Geometry check sheet. Reference: the model listing, model coordinates, mm. A direction names the side the tool comes from. Round coordinates to 2 decimals unless told otherwise and drop trailing zeros. Loops run counter-clockwise (first coordinate to the right, second up) from the corner with the lowest first, then second, coordinate; pieces in that order, holes last.
```python
from build123d import *

# Parameters (mm, degrees)
SKETCH_2_W      = 200
SKETCH_2_H      = 200
SKETCH_2_R      = 1.6
SKETCH_2_R_2    = 3
SKETCH_2_W_2    = 3
SKETCH_2_H_2    = 40
EXTRUDE_1_DEPTH = 3
FILLET_2_R      = 20


with BuildPart() as part:
    # 草图2 → 凸台-拉伸1 (new body)
    with BuildSketch(Plane(origin=(0, 0, 0), x_dir=(1, 0, 0), z_dir=(0, 1, 0))):
        Rectangle(SKETCH_2_W, SKETCH_2_H)
        with Locations(Location((-52.5, 52.5, 0), (0, 0, 270))):
            Circle(SKETCH_2_R, mode=Mode.SUBTRACT)
        with Locations(Location((-45.428932188, 45.428932188, 0), (0, 0, 270))):
            Circle(SKETCH_2_R, mode=Mode.SUBTRACT)
        with Locations(Location((-38.357864376, 38.357864376, 0), (0, 0, 270))):
            Circle(SKETCH_2_R, mode=Mode.SUBTRACT)
        with Locations(Location((52.5, 52.5, 0), (0, 0, 270))):
            Circle(SKETCH_2_R, mode=Mode.SUBTRACT)
        with Locations(Location((45.428932188, 45.428932188, 0), (0, 0, 270))):
            Circle(SKETCH_2_R, mode=Mode.SUBTRACT)
        with Locations(Location((38.357864376, 38.357864376, 0), (0, 0, 270))):
            Circle(SKETCH_2_R, mode=Mode.SUBTRACT)
        with Locations(Location((52.5, -52.5, 0), (0, 0, 270))):
            Circle(SKETCH_2_R, mode=Mode.SUBTRACT)
        with Locations(Location((45.428932188, -45.428932188, 0), (0, 0, 270))):
            Circle(SKETCH_2_R, mode=Mode.SUBTRACT)
        with Locations(Location((38.357864376, -38.357864376, 0), (0, 0, 270))):
            Circle(SKETCH_2_R, mode=Mode.SUBTRACT)
        with Locations(Location((-52.5, -52.5, 0), (0, 0, 270))):
            Circle(SKETCH_2_R, mode=Mode.SUBTRACT)
        with Locations(Location((-45.428932188, -45.428932188, 0), (0, 0, 270))):
            Circle(SKETCH_2_R, mode=Mode.SUBTRACT)
        with Locations(Location((-38.357864376, -38.357864376, 0), (0, 0, 270))):
            Circle(SKETCH_2_R, mode=Mode.SUBTRACT)
        with Locations(Location((0, 0, 0), (0, 0, 270))):
            Circle(SKETCH_2_R_2, mode=Mode.SUBTRACT)
        with BuildLine():
            Line((-60, 73.5), (60, 73.5))
            ThreePointArc((60, 73.5), (69, 82.5), (60, 91.5))
            Line((60, 91.5), (-60, 91.5))
            ThreePointArc((-60, 91.5), (-69, 82.5), (-60, 73.5))
        make_face(mode=Mode.SUBTRACT)
        with BuildLine():
            Line((-60, -73.5), (60, -73.5))
            ThreePointArc((60, -73.5), (69, -82.5), (60, -91.5))
            Line((60, -91.5), (-60, -91.5))
            ThreePointArc((-60, -91.5), (-69, -82.5), (-60, -73.5))
        make_face(mode=Mode.SUBTRACT)
        with Locations((74.942911166, 65)):
            Rectangle(SKETCH_2_W_2, SKETCH_2_H_2, mode=Mode.SUBTRACT)
        with Locations((87.942911166, 65)):
            Rectangle(SKETCH_2_W_2, SKETCH_2_H_2, mode=Mode.SUBTRACT)
        with Locations((74.942911166, -65)):
            Rectangle(SKETCH_2_W_2, SKETCH_2_H_2, mode=Mode.SUBTRACT)
        with Locations((87.942911166, -65)):
            Rectangle(SKETCH_2_W_2, SKETCH_2_H_2, mode=Mode.SUBTRACT)
        with Locations((-74.942911166, -65)):
            Rectangle(SKETCH_2_W_2, SKETCH_2_H_2, mode=Mode.SUBTRACT)
        with Locations((-87.942911166, -65)):
            Rectangle(SKETCH_2_W_2, SKETCH_2_H_2, mode=Mode.SUBTRACT)
        with Locations((-87.942911166, 65)):
            Rectangle(SKETCH_2_W_2, SKETCH_2_H_2, mode=Mode.SUBTRACT)
        with Locations((-74.942911166, 65)):
            Rectangle(SKETCH_2_W_2, SKETCH_2_H_2, mode=Mode.SUBTRACT)
        with BuildLine():
            Line((22.714466094, 23.428932188), (-22.714466094, 23.428932188))
            ThreePointArc((-22.714466094, 23.428932188), (-26.714466094, 27.428932188), (-22.714466094, 31.428932188))
            Line((-22.714466094, 31.428932188), (22.714466094, 31.428932188))
            ThreePointArc((22.714466094, 31.428932188), (26.714466094, 27.428932188), (22.714466094, 23.428932188))
        make_face(mode=Mode.SUBTRACT)
        with BuildLine():
            Line((22.714466094, 41.428932188), (-22.714466094, 41.428932188))
            ThreePointArc((-22.714466094, 41.428932188), (-26.714466094, 45.428932188), (-22.714466094, 49.428932188))
            Line((-22.714466094, 49.428932188), (22.714466094, 49.428932188))
            ThreePointArc((22.714466094, 49.428932188), (26.714466094, 45.428932188), (22.714466094, 41.428932188))
        make_face(mode=Mode.SUBTRACT)
        with BuildLine():
            Line((22.714466094, 59.428932188), (-22.714466094, 59.428932188))
            ThreePointArc((-22.714466094, 59.428932188), (-26.714466094, 63.428932188), (-22.714466094, 67.428932188))
            Line((-22.714466094, 67.428932188), (22.714466094, 67.428932188))
            ThreePointArc((22.714466094, 67.428932188), (26.714466094, 63.428932188), (22.714466094, 59.428932188))
        make_face(mode=Mode.SUBTRACT)
        with BuildLine():
            Line((22.714466094, -23.428932188), (-22.714466094, -23.428932188))
            ThreePointArc((-22.714466094, -23.428932188), (-26.714466094, -27.428932188), (-22.714466094, -31.428932188))
            Line((-22.714466094, -31.428932188), (22.714466094, -31.428932188))
            ThreePointArc((22.714466094, -31.428932188), (26.714466094, -27.428932188), (22.714466094, -23.428932188))
        make_face(mode=Mode.SUBTRACT)
        with BuildLine():
            Line((22.714466094, -41.428932188), (-22.714466094, -41.428932188))
            ThreePointArc((-22.714466094, -41.428932188), (-26.714466094, -45.428932188), (-22.714466094, -49.428932188))
            Line((-22.714466094, -49.428932188), (22.714466094, -49.428932188))
            ThreePointArc((22.714466094, -49.428932188), (26.714466094, -45.428932188), (22.714466094, -41.428932188))
        make_face(mode=Mode.SUBTRACT)
        with BuildLine():
            Line((22.714466094, -59.428932188), (-22.714466094, -59.428932188))
            ThreePointArc((-22.714466094, -59.428932188), (-26.714466094, -63.428932188), (-22.714466094, -67.428932188))
            Line((-22.714466094, -67.428932188), (22.714466094, -67.428932188))
            ThreePointArc((22.714466094, -67.428932188), (26.714466094, -63.428932188), (22.714466094, -59.428932188))
        make_face(mode=Mode.SUBTRACT)
        with BuildLine():
            Line((22.5, -12.5), (22.5, 12.5))
            ThreePointArc((22.5, 12.5), (25, 15), (27.5, 12.5))
            Line((27.5, 12.5), (27.5, -12.5))
            ThreePointArc((27.5, -12.5), (25, -15), (22.5, -12.5))
        make_face(mode=Mode.SUBTRACT)
        with BuildLine():
            Line((32.5, -17.5), (32.5, 17.5))
            ThreePointArc((32.5, 17.5), (35, 20), (37.5, 17.5))
            Line((37.5, 17.5), (37.5, -17.5))
            ThreePointArc((37.5, -17.5), (35, -20), (32.5, -17.5))
        make_face(mode=Mode.SUBTRACT)
        with BuildLine():
            Line((42.5, -22.5), (42.5, 22.5))
            ThreePointArc((42.5, 22.5), (45, 25), (47.5, 22.5))
            Line((47.5, 22.5), (47.5, -22.5))
            ThreePointArc((47.5, -22.5), (45, -25), (42.5, -22.5))
        make_face(mode=Mode.SUBTRACT)
        with BuildLine():
            Line((52.5, -27.5), (52.5, 27.5))
            ThreePointArc((52.5, 27.5), (55, 30), (57.5, 27.5))
            Line((57.5, 27.5), (57.5, -27.5))
            ThreePointArc((57.5, -27.5), (55, -30), (52.5, -27.5))
        make_face(mode=Mode.SUBTRACT)
        with BuildLine():
            Line((62.5, -32.5), (62.5, 32.5))
            ThreePointArc((62.5, 32.5), (65, 35), (67.5, 32.5))
            Line((67.5, 32.5), (67.5, -32.5))
            ThreePointArc((67.5, -32.5), (65, -35), (62.5, -32.5))
        make_face(mode=Mode.SUBTRACT)
        with BuildLine():
            Line((-22.5, -12.5), (-22.5, 12.5))
            ThreePointArc((-22.5, 12.5), (-25, 15), (-27.5, 12.5))
            Line((-27.5, 12.5), (-27.5, -12.5))
            ThreePointArc((-27.5, -12.5), (-25, -15), (-22.5, -12.5))
        make_face(mode=Mode.SUBTRACT)
        with BuildLine():
            Line((-32.5, -17.5), (-32.5, 17.5))
            ThreePointArc((-32.5, 17.5), (-35, 20), (-37.5, 17.5))
            Line((-37.5, 17.5), (-37.5, -17.5))
            ThreePointArc((-37.5, -17.5), (-35, -20), (-32.5, -17.5))
        make_face(mode=Mode.SUBTRACT)
        with BuildLine():
            Line((-42.5, -22.5), (-42.5, 22.5))
            ThreePointArc((-42.5, 22.5), (-45, 25), (-47.5, 22.5))
            Line((-47.5, 22.5), (-47.5, -22.5))
            ThreePointArc((-47.5, -22.5), (-45, -25), (-42.5, -22.5))
        make_face(mode=Mode.SUBTRACT)
        with BuildLine():
            Line((-52.5, -27.5), (-52.5, 27.5))
            ThreePointArc((-52.5, 27.5), (-55, 30), (-57.5, 27.5))
            Line((-57.5, 27.5), (-57.5, -27.5))
            ThreePointArc((-57.5, -27.5), (-55, -30), (-52.5, -27.5))
        make_face(mode=Mode.SUBTRACT)
        with BuildLine():
            Line((-62.5, -32.5), (-62.5, 32.5))
            ThreePointArc((-62.5, 32.5), (-65, 35), (-67.5, 32.5))
            Line((-67.5, 32.5), (-67.5, -32.5))
            ThreePointArc((-67.5, -32.5), (-65, -35), (-62.5, -32.5))
        make_face(mode=Mode.SUBTRACT)
        with BuildLine():
            Line((88.942911166, 30), (88.942911166, -30))
            ThreePointArc((88.942911166, -30), (81.442911166, -37.5), (73.942911166, -30))
            Line((73.942911166, -30), (73.942911166, 30))
            ThreePointArc((73.942911166, 30), (81.442911166, 37.5), (88.942911166, 30))
        make_face(mode=Mode.SUBTRACT)
        with BuildLine():
            Line((-88.942911166, 30), (-88.942911166, -30))
            ThreePointArc((-88.942911166, -30), (-81.442911166, -37.5), (-73.942911166, -30))
            Line((-73.942911166, -30), (-73.942911166, 30))
            ThreePointArc((-73.942911166, 30), (-81.442911166, 37.5), (-88.942911166, 30))
        make_face(mode=Mode.SUBTRACT)
    extrude(amount=EXTRUDE_1_DEPTH)

    # 圆角2
    fillet_2_edges = [part.edges().sort_by_distance(p)[0] for p in [
        (-100, 1.5, -100),
        (100, 1.5, -100),
        (100, 1.5, 100),
        (-100, 1.5, 100),
    ]]
    fillet(fillet_2_edges, radius=FILLET_2_R)


solid = part.part
```
1) Sectioned sample at B-B, the plane z = 0. State how many separate pieces and enclosed holes the cut face has, then the cut area to 3 significant figures.
Report:
separate pieces: 14
enclosed holes: 0
area: 342 mm2
2) Sectioned sample at A-A, the plane x = -65. Record the cut outline in (y, z).
Report:
outline: (0, -100) - (3, -100) - (3, -89.98) - (0, -89.98) - close; (0, -75.02) - (3, -75.02) - (3, -35) - (0, -35) - close; (0, 35) - (3, 35) - (3, 75.02) - (0, 75.02) - close; (0, 89.98) - (3, 89.98) - (3, 100) - (0, 100) - close
3) Access from +Z, -Z, +X, -X, +Y, -Y to the whole of each face (thin tool, end or side, straight path). Record for faces 1 (the face through (-94.297, 1.521, 93.986)), 2 (the face through (68.998, 1.479, 82.302)).
Report:
face 1: +Z, -X, +Y, -Y
face 2: +Y, -Y
4) Mould release check, pull along X, two halves, no side actions. Record for faces 3 (the face through (-24, 3, 21)), 4 (the face through (68.998, 1.479, -82.302)), 5 (the face through (93.986, 1.521, -94.297)): +X half, -X half, draft (parallel to the pull), parting line (faces both ways), or undercut.
Report:
face 3: draft
face 4: undercut
face 5: +X half
5) Gauge pin test, flat end, axial feed: pin 1 (1.5 mm diameter, centred on x = -88, y = 1.5, fed in from +Z). Record the tip position at first contact, or that the pin passes through.
Report:
pin 1: stops at z = 98.64
6) Scan lines: line 1 along Z through (x, y) = (49.5, 2.15); line 2 along X through (y, z) = (2.25, 67); line 3 along X through (y, z) = (1.35, 66). Record each from-to range of solid material in increasing order.
Report:
line 1: z = -100 to -91.5, -73.5 to 73.5, 91.5 to 100
line 2: x = -100 to -89.44, -86.44 to -76.44, -73.44 to -24.52, 24.52 to 73.44, 76.44 to 86.44, 89.44 to 100
line 3: x = -100 to -89.44, -86.44 to -76.44, -73.44 to -25.78, 25.78 to 73.44, 76.44 to 86.44, 89.44 to 100
